Geometry: final body of the model. Coordinates: model frame, mm. Face numbers are marked on the shaded views. A direction names the side the tool comes from. Coordinates: 2 decimals unless noted, no trailing zeros. Loops run counter-clockwise (first coordinate to the right, second up) from the corner with the lowest first, then second, coordinate; pieces in that order, holes last. Notation, with made-up numbers: (31.25, -5.5) - (48.25, -5.5) arc R29 cw to (48.25, 23.5) - close; hole circle Ø10 at (79.25, 8.25). An arc over 180 degrees is marked (long way). Answer in a Markdown table with one row per item.
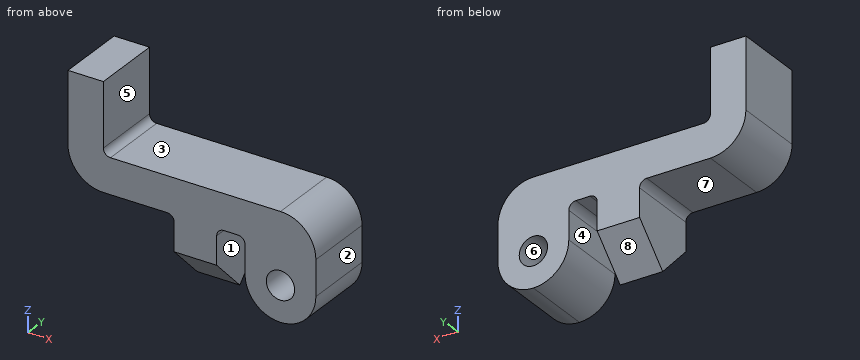
from build123d import *

# Parameters (mm, degrees)
F0_R     = 2
F1_DEPTH = 10
F2_R     = 1
F4_DEPTH = 6


with BuildPart() as f1:
    # F0 (on Front) → F1 (new body)
    with BuildSketch(Plane.XZ):
        with BuildLine():
            Line((5, 18.538928), (0, 18.538928))
            Line((0, 18.538928), (0, 8.538928))
            ThreePointArc((0, 8.538928), (1.464466, 5.003394), (5, 3.538928))
            Line((5, 3.538928), (14, 3.538928))
            ThreePointArc((14, 3.538928), (14.707107, 3.246035), (15, 2.538928))
            Line((15, 2.538928), (15, -6.461072))
            Line((15, -6.461072), (21, -6.461072))
            Line((21, -6.461072), (21, 2.538928))
            ThreePointArc((21, 2.538928), (21.292893, 3.246035), (22, 3.538928))
            Line((22, 3.538928), (24, 3.538928))
            ThreePointArc((24, 3.538928), (24.707107, 3.246035), (25, 2.538928))
            Line((25, 2.538928), (25, -1.461072))
            ThreePointArc((25, -1.461072), (26.464466, -4.996606), (30, -6.461072))
            ThreePointArc((30, -6.461072), (33.535534, -4.996606), (35, -1.461072))
            Line((35, -1.461072), (35, 3.538928))
            ThreePointArc((35, 3.538928), (33.535534, 7.074462), (30, 8.538928))
            Line((30, 8.538928), (5, 8.538928))
            Line((5, 8.538928), (5, 18.538928))
        make_face()
        with Locations((30, -1.461072)):
            Circle(F0_R, mode=Mode.SUBTRACT)
    extrude(amount=F1_DEPTH)

    # F2
    f2_edges = [f1.edges().sort_by_distance(p)[0] for p in [
        (5, -5, 8.538928),
    ]]
    fillet(f2_edges, radius=F2_R)

    # F3 (on face) → F4 (cut)
    with BuildSketch(Plane(origin=(15, 0, 0), x_dir=(0, -1, 0), z_dir=(-1, 0, 0))):
        Polygon((0, -6.461072), (5, -6.461072), (0, -1.461072), align=None)
        Polygon((10, -1.461072), (5, -6.461072), (10, -6.461072), align=None)
    extrude(amount=-F4_DEPTH, mode=Mode.SUBTRACT)


solid = f1.part
(1) Cut plane A-A on y = -8.75. Output: boundary loops of the cut face in (x, z), then the cut area to 3 significant figures.
Verdict:
| item | result |
|---|---|
| outline | (0, 8.54) arc R5 ccw to (5, 3.54) - (14, 3.54) arc R1 cw to (15, 2.54) - (15, -2.71) - (21, -2.71) - (21, 2.54) arc R1 cw to (22, 3.54) - (24, 3.54) arc R1 cw to (25, 2.54) - (25, -1.46) arc R5 ccw to (35, -1.46) - (35, 3.54) arc R5 ccw to (30, 8.54) - (6, 8.54) arc R1 cw to (5, 9.54) - (5, 18.54) - (0, 18.54) - close; hole circle Ø4 at (30, -1.46) |
| area | 329 mm² |
(2) Cut plane B-B on x = 29. Output: boundary loops of the cut face in (y, z), then the cut area to 3 significant figures.
Verdict:
| item | result |
|---|---|
| outline | (-10, -6.36) - (0, -6.36) - (0, -3.19) - (-10, -3.19) - close; (-10, 0.27) - (0, 0.27) - (0, 8.54) - (-10, 8.54) - close |
| area | 114 mm² |
(3) Pull-direction query (X, two-part tool) for the marked faces 1, 2 and 3; classes: pulls with the +X half, pulls with the -X half, needs draft (parallel to the pull), parting line crosses it, or undercut.
Verdict:
| item | result |
|---|---|
| face 1 | undercut |
| face 2 | pulls with the +X half |
| face 3 | needs draft |
(4) Cut plane D-D on z = 13.25. Output: boundary loops of the cut face in (x, y), then the cut area to 3 significant figures.
Verdict:
| item | result |
|---|---|
| outline | (0, -10) - (5, -10) - (5, 0) - (0, 0) - close |
| area | 50.0 mm² |
(5) Cut plane C-C on x = 15.5. Output: boundary loops of the cut face in (y, z), then the cut area to 3 significant figures.
Verdict:
| item | result |
|---|---|
| outline | (-10, -1.46) - (-5, -6.46) - (0, -1.46) - (0, 8.54) - (-10, 8.54) - close |
| area | 125 mm² |
(6) Access query for the marked faces 4, 5, 6, 7 and 8. Directions: +Z, -Z, +X, -X, +Y, -Y. A direction counts if a zero-diameter tool reaches every point of the face in a straight line with its end or side. Return the directions, or none.
Verdict:
| item | result |
|---|---|
| face 4 | -Z, +Y, -Y |
| face 5 | +Z, +X, +Y, -Y |
| face 6 | +Y, -Y |
| face 7 | -Z, -X, +Y, -Y |
| face 8 | -Z, -X, +Y |
(7) First-contact query: pin 1 Ø4.5 at (x, z) = (30, -1.46) entering from -Y; pin 2 Ø1 at (x, y) = (23.5, -6) entering from -Z; pin 3 Ø2.5 at (y, z) = (-5, -3) entering from +X; pin 4 Ø6 at (x, z) = (9, -1.5) entering from -Y. Flat tips, straight axial feed; report the tip coordinate or a pass-through.
Verdict:
| item | result |
|---|---|
| pin 1 | stops at y = -10 |
| pin 2 | stops at z = 3.54 |
| pin 3 | stops at x = 34.99 |
| pin 4 | passes through |
(8) Ray query, probe 1 along X at (y, z) = (-9.5, -1); probe 2 along Z at (x, y) = (30, -4.5); probe 3 along Z at (x, y) = (6.5, -4.5). Return the intervals inside material, ascending.
Verdict:
| item | result |
|---|---|
| probe 1 | x = 15 to 21, 25 to 28.05, 31.95 to 35 |
| probe 2 | z = -6.46 to -3.46, 0.54 to 8.54 |
| probe 3 | z = 3.54 to 8.54 |
